Solid Edge part; units mm, degrees
sketch "Sketch1" plane through (0, 0, 0) normal (0, 0, 1) x (1, 0, 0)
  circle A0 centre (0, 0) radius 35
extrude "Protrusion1" add sketch "Sketch1" along normal blind 7
sketch "Sketch2" plane through (0, 0, 7) normal (0, 0, 1) x (1, 0, 0)
  line L0 (-17.5, -17.5) -> (17.5, -17.5)
  line L1 (17.5, -17.5) -> (17.5, 17.5)
  line L2 (17.5, 17.5) -> (-17.5, 17.5)
  line L3 (-17.5, 17.5) -> (-17.5, -17.5)
  dimension "D1" = 17.5
extrude "ExtrudedProtrusion_2" add sketch "Sketch2" along normal blind 63
sketch "Sketch3" plane through (0, 0, 70) normal (0, 0, 1) x (1, 0, 0)
  line L0 (-67.8, -24.7487) -> (24.7487, -24.7487)
  line L1 (24.7487, -24.7487) -> (24.7487, 24.7487)
  line L2 (24.7487, 24.7487) -> (-67.8, 24.7487)
  line L3 (-67.8, 24.7487) -> (-67.8, -24.7487)
  dimension "D1" = 24.7487
extrude "ExtrudedProtrusion_3" add sketch "Sketch3" along normal blind 7
sketch "Sketch4" plane through (-67.8, 0, 73.5) normal (-1, 0, 0) x (0, -1, 0)
  line L0 (-60, 3.5) -> (60, 3.5)
  line L1 (60, 3.5) -> (60, 100.35)
  line L2 (60, 100.35) -> (-60, 100.35)
  line L3 (-60, 100.35) -> (-60, 3.5)
  dimension "D1" = 60
extrude "ExtrudedProtrusion_4" add sketch "Sketch4" against normal blind 7
sketch "Sketch5" plane through (-60.8, 0, 125.425) normal (1, 0, 0) x (0, 1, 0)
  line L0 (-50, 39.775) -> (50, 39.775)
  line L1 (50, 37.075) -> (-50, 37.075)
  arc A0 (-50, 37.075) -> (-50, 39.775) centre (-50, 38.425) cw
  arc A1 (50, 39.775) -> (50, 37.075) centre (50, 38.425) cw
  dimension "D1" = 50
extrude "ExtrudedProtrusion_5" add sketch "Sketch5" along normal blind 90
Verification items for the finished model (mm, model axes). A direction names the side the tool comes from. Give positions to 0.01 mm unless a question says otherwise; leave off trailing zeros. Write each loop counter-clockwise with the first axis right and the second up, starting at its lowest first coordinate (ties: lowest second). Pieces come first, ordered by that corner, then holes.
(1) Access from +Z, -Z, +X, -X, +Y, -Y to the whole of each face (thin tool, end or side, straight path). Record for faces 4 (the face through (-21, 24.749, 73)), 5 (the face through (-19, 0, 77)), 6 (the face through (-22, -24.749, 73)).
(2) Cross-section at D-D (y = -21.5). Enter the section's corners in (x, z), plus the area to 3 significant figures.
(3) Mould release check, pull along Z, two halves, no side actions. Record for faces 1 (the face through (-64, 43, 77)), 2 (the face through (-64, -1, 173.85)), 3 (the face through (-60.8, -1, 126)): +Z half, -Z half, draft (parallel to the pull), parting line (faces both ways), or undercut.
(4) Gauge pin test, flat ends, axial feed: pin 1 (2 mm diameter, centred on y = 3.5, z = 74, fed in from +X); pin 2 (2 mm diameter, centred on y = 16.5, z = 126, fed in from +X); pin 3 (5 mm diameter, centred on x = -18.5, y = -30.5, fed in from +Z). Record the tip position at first contact, or that the pin passes through.
(5) Cross-section at B-B (y = -41). Enter the section's corners in (x, z), plus the area to 3 significant figures.
(6) Cross-section at A-A (x = 0). Enter the section's corners in (y, z).
(7) Cross-section at C-C (x = -50.5). Enter the section's corners in (y, z).
(8) Material ranges on line 1 (Z direction, x = -32.5, y = -23); line 2 (Z direction, x = -11, y = -19); line 3 (X direction, y = 46, z = 148.5), recorded low to high.
Worked out:
1. face 4: +X, -X, +Y
1. face 5: +X, +Y, -Y
1. face 6: +X, -X, -Y
2. outline: (-67.8, 70) - (24.75, 70) - (24.75, 77) - (-60.8, 77) - (-60.8, 162.5) - (29.2, 162.5) - (29.2, 165.2) - (-60.8, 165.2) - (-60.8, 173.85) - (-67.8, 173.85) - close; (-27.62, 0) - (27.62, 0) - (27.62, 7) - (-27.62, 7) - close
2. area: 1,960 mm2
3. face 1: -Z half
3. face 2: +Z half
3. face 3: undercut
4. pin 1: stops at x = 24.75
4. pin 2: stops at x = -60.8
4. pin 3: stops at z = 165.2
5. outline: (-67.8, 77) - (-60.8, 77) - (-60.8, 162.5) - (29.2, 162.5) - (29.2, 165.2) - (-60.8, 165.2) - (-60.8, 173.85) - (-67.8, 173.85) - close
5. area: 921 mm2
6. outline: (-50, 162.5) - (50, 162.5) arc R1.35 ccw to (50, 165.2) - (-50, 165.2) arc R1.35 ccw to start; (-35, 0) - (35, 0) - (35, 7) - (17.5, 7) - (17.5, 70) - (24.75, 70) - (24.75, 77) - (-24.75, 77) - (-24.75, 70) - (-17.5, 70) - (-17.5, 7) - (-35, 7) - close
7. outline: (-50, 162.5) - (50, 162.5) arc R1.35 ccw to (50, 165.2) - (-50, 165.2) arc R1.35 ccw to start; (-24.75, 70) - (24.75, 70) - (24.75, 77) - (-24.75, 77) - close
8. line 1: z = 70 to 77, 162.5 to 165.2
8. line 2: z = 0 to 7, 70 to 77, 162.5 to 165.2
8. line 3: x = -67.8 to -60.8
